from build123d import *

# Parameters (mm, degrees)
SKETCH1_W               = 38
SKETCH1_H               = 54
PCB_DEPTH               = 1.5
ATMEGA_DEPTH            = 1
SKETCH3_W               = 7.3
SKETCH3_H               = 5.5
SKETCH3_W_2             = 6.5
SKETCH3_H_2             = 6.5
USB_AND_RST_DEPTH       = 2
SKETCH4_R               = 1.5
BUTTON_DEPTH            = 0.5
CUT_EXTRUDE1_DEPTH      = 34.109666262
CUT_EXTRUDE1_DEPTH_BACK = 34.109666262
SKETCH5_R               = 1.5


with BuildPart() as part:
    # Sketch1 → PCB (new body)
    with BuildSketch(Plane(origin=(0, 0, 0), x_dir=(1, 0, 0), z_dir=(0, 1, 0))):
        Rectangle(SKETCH1_W, SKETCH1_H)
    extrude(amount=PCB_DEPTH)

    # Sketch2 → ATMega (add)
    with BuildSketch(Plane(origin=(0, 1.5, 0), x_dir=(1, 0, 0), z_dir=(0, 1, 0))):
        Polygon((0, -0.266695552), (9.616652224, -9.883347776), (0, -19.5), (-9.616652224, -9.883347776), align=None)
    extrude(amount=ATMEGA_DEPTH)

    # Sketch3 → USB and RST (add)
    with BuildSketch(Plane(origin=(0, 1.5, 0), x_dir=(1, 0, 0), z_dir=(0, 1, 0))):
        with Locations((5.85, 24.25)):
            Rectangle(SKETCH3_W, SKETCH3_H)
        with Locations((15.75, 21.75)):
            Rectangle(SKETCH3_W_2, SKETCH3_H_2)
    extrude(amount=USB_AND_RST_DEPTH)

    # Sketch4 → Button (add)
    with BuildSketch(Plane(origin=(0, 3.5, 0), x_dir=(1, 0, 0), z_dir=(0, 1, 0))):
        with Locations(Location((15.75, 21.75, 0), (0, 0, 270))):
            Circle(SKETCH4_R)
    extrude(amount=BUTTON_DEPTH)

    # Sketch5 → Cut-Extrude1 (cut, two sides: drawn at the far end of the back side and taken through both)
    with BuildSketch(Plane(origin=(0, 1.5, 0), x_dir=(1, 0, 0), z_dir=(0, 1, 0)).offset(-CUT_EXTRUDE1_DEPTH_BACK)):
        with Locations(Location((11, 14, 0), (0, 0, 270))):
            Circle(SKETCH5_R)
        with Locations(Location((4, -24, 0), (0, 0, 270))):
            Circle(SKETCH5_R)
    extrude(amount=CUT_EXTRUDE1_DEPTH + CUT_EXTRUDE1_DEPTH_BACK, mode=Mode.SUBTRACT)


solid = part.part
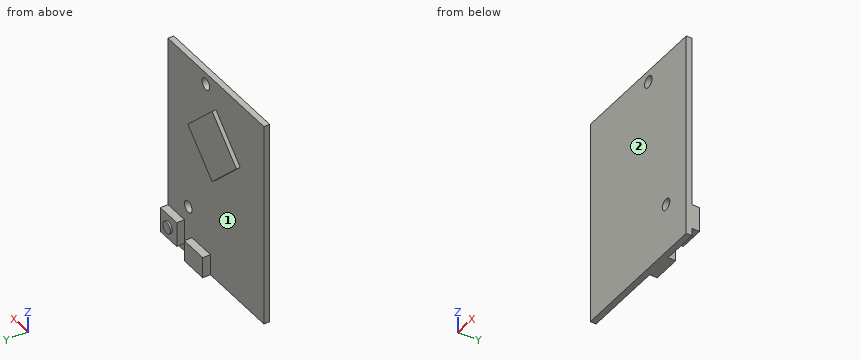
Input: part model. Units: mm. Frame: model coordinates. Face numbers are marked on the shaded views. Give positions to 0.01 mm unless a question says otherwise; leave off trailing zeros. Order: outer loops, then holes, each group sorted by start corner. A loop starts at its lowest first (then second) coordinate and runs counter-clockwise, first axis right, second up. Notation, with made-up numbers: (38, 16) - (90, 16) arc R15 cw to (90, 36) - close; hole circle Ø6 at (54.5, 12). An arc over 180 degrees is marked (long way). Answer as a JSON object with one key per item and string values. Group by question number.
Q1. First-contact query: pin 1 Ø2.5 at (x, z) = (11, -14) entering from +Y; pin 2 Ø1 at (x, y) = (5.5, 2.5) entering from +Z; pin 3 Ø15.5 at (x, z) = (-3, 13) entering from +Y; pin 4 Ø3 at (x, z) = (5.5, -23.5) entering from +Y. Flat tips, straight axial feed; report the tip coordinate or a pass-through.
Q2. Cut plane C-C, the plane z = 17. Output: boundary loops of the cut face in (x, y).
Q3. Cut plane B-B, the plane z = 24. Output: boundary loops of the cut face in (x, y), then the cut area to 3 significant figures.
Q4. Cut plane A-A, the plane x = 11. Output: boundary loops of the cut face in (y, z), then the cut area to 3 significant figures.
Q5. Cut plane D-D, the plane x = 15.75. Output: boundary loops of the cut face in (y, z).
Q6. Mould query, pull axis Z, two halves, no side actions, for the marked faces 1 and 2. Classes: pulls with the +Z half, pulls with the -Z half, needs draft (parallel to the pull), parting line crosses it, or undercut.
Q7. Line query: probe 1 along X at (y, z) = (0.95, -14); probe 2 along X at (y, z) = (1.05, 24); probe 3 along Z at (x, y) = (4, 0.9). Output: solid intervals per line, ascending.
Results:
{
 "1": {"pin 1": "through", "pin 2": "z = 14.5", "pin 3": "y = 2.5", "pin 4": "y = 3.5"},
 "2": {"outline": "(-19, 0) - (19, 0) - (19, 1.5) - (2.5, 1.5) - (2.5, 2.5) - (-2.5, 2.5) - (-2.5, 1.5) - (-19, 1.5) - close"},
 "3": {"outline": "(-19, 0) - (2.5, 0) - (2.5, 1.5) - (-19, 1.5) - close; (5.5, 0) - (19, 0) - (19, 1.5) - (5.5, 1.5) - close", "area": "52.5 mm^2"},
 "4": {"outline": "(0, -27) - (1.5, -27) - (1.5, -15.5) - (0, -15.5) - close; (0, -12.5) - (1.5, -12.5) - (1.5, 27) - (0, 27) - close", "area": "76.5 mm^2"},
 "5": {"outline": "(0, -27) - (1.5, -27) - (1.5, -25) - (3.5, -25) - (3.5, -23.25) - (4, -23.25) - (4, -20.25) - (3.5, -20.25) - (3.5, -18.5) - (1.5, -18.5) - (1.5, 27) - (0, 27) - close"},
 "6": {"face 1": "undercut", "face 2": "needs draft"},
 "7": {"probe 1": "-19 to 9.5, 12.5 to 19", "probe 2": "-19 to 2.5, 5.5 to 19", "probe 3": "-27 to 22.5, 25.5 to 27"}
}
